from build123d import *

# Parameters (mm, degrees)
SKETCH1_W           = 42.3
SKETCH1_H           = 42
BOSS_EXTRUDE1_DEPTH = 38
SKETCH2_R           = 2.5
BOSS_EXTRUDE2_DEPTH = 19
SKETCH3_R           = 1.5
CUT_EXTRUDE1_DEPTH  = 4.5


with BuildPart() as part:
    # Sketch1 → Boss-Extrude1 (new body)
    with BuildSketch(Plane(origin=(0, 0, 0), x_dir=(1, 0, 0), z_dir=(0, 1, 0))):
        Rectangle(SKETCH1_W, SKETCH1_H)
    extrude(amount=BOSS_EXTRUDE1_DEPTH)

    # Sketch2 → Boss-Extrude2 (add)
    with BuildSketch(Plane(origin=(0, 38, 0), x_dir=(1, 0, 0), z_dir=(0, 1, 0))):
        Circle(SKETCH2_R)
    extrude(amount=BOSS_EXTRUDE2_DEPTH)

    # Sketch3 → Cut-Extrude1 (cut)
    with BuildSketch(Plane(origin=(0, 38, 0), x_dir=(1, 0, 0), z_dir=(0, 1, 0))):
        with Locations((-15.5, 15.5)):
            Circle(SKETCH3_R)
        with Locations((15.5, 15.5)):
            Circle(SKETCH3_R)
        with Locations((15.5, -15.5)):
            Circle(SKETCH3_R)
        with Locations((-15.5, -15.5)):
            Circle(SKETCH3_R)
    extrude(amount=-CUT_EXTRUDE1_DEPTH, mode=Mode.SUBTRACT)


solid = part.part
Here's how the part is built. I have some questions about the finished solid (model axes, mm). A direction names the side the tool comes from. Coordinates: 2 decimals unless noted, no trailing zeros. Write each loop counter-clockwise with the first axis right and the second up, starting at its lowest first coordinate (ties: lowest second). Pieces come first, ordered by that corner, then holes.
1) If we section it at B-B (x = 0): List the corners of the cut face in (y, z) for me, plus the area to 3 significant figures.
Filled in:
outline: (0, -21) - (38, -21) - (38, -2.5) - (57, -2.5) - (57, 2.5) - (38, 2.5) - (38, 21) - (0, 21) - close
area: 1,690 mm2
2) I'm going to push flat-ended pins straight in: pin 1 (4 mm diameter, centred on x = 12, z = 5, fed in from +Y); pin 2 (1.8 mm diameter, centred on x = 15.5, z = 15.5, fed in from +Y). Where does each tip first touch, or does it pass through?
Filled in:
pin 1: stops at y = 38
pin 2: stops at y = 33.5
3) Which directions (+Z, -Z, +X, -X, +Y, -Y) give clear straight access to the entire face, cutting with the end or side of a thin tool? Please do faces 1 (the face through (15, 33.5, -16)), 2 (the face through (0, 57, 0)).
Filled in:
face 1: +Y
face 2: +Z, -Z, +X, -X, +Y
4) If we section it at C-C (x = 15.5): List the corners of the cut face in (y, z) for me, plus the area to 3 significant figures.
Filled in:
outline: (0, -21) - (38, -21) - (38, -17) - (33.5, -17) - (33.5, -14) - (38, -14) - (38, 14) - (33.5, 14) - (33.5, 17) - (38, 17) - (38, 21) - (0, 21) - close
area: 1,570 mm2
5) If we section it at D-D (z = 0): List the corners of the cut face in (x, y) for me.
Filled in:
outline: (-21.15, 0) - (21.15, 0) - (21.15, 38) - (2.5, 38) - (2.5, 57) - (-2.5, 57) - (-2.5, 38) - (-21.15, 38) - close
6) If I drill on line 1 (Z direction, x = -15.5, y = 36); line 2 (X direction, y = 35, z = 15); line 3 (Z direction, x = -15, y = 36), over which ranges is the centre line in solid material (lowest first)?
Filled in:
line 1: z = -21 to -17, -14 to 14, 17 to 21
line 2: x = -21.15 to -16.91, -14.09 to 14.09, 16.91 to 21.15
line 3: z = -21 to -16.91, -14.09 to 14.09, 16.91 to 21
7) Thinking about a two-plate mould opening in Z: for faces 3 (the face through (0, 38, -5)), 4 (the face through (0, 19, 21)), 5 (the face through (-16, 33.5, 15)), which applies, +Z half, -Z half, draft (parallel to the pull), parting line (faces both ways), or undercut?
Filled in:
face 3: draft
face 4: +Z half
face 5: undercut
8) If we section it at A-A (z = -15.5): List the corners of the cut face in (x, y) for me.
Filled in:
outline: (-21.15, 0) - (21.15, 0) - (21.15, 38) - (17, 38) - (17, 33.5) - (14, 33.5) - (14, 38) - (-14, 38) - (-14, 33.5) - (-17, 33.5) - (-17, 38) - (-21.15, 38) - close
